For this review, take the finished solid that the model builds, in its own axes (mm). Face numbers are marked on the shaded views. A direction names the side the tool comes from. Coordinates: 2 decimals unless noted, no trailing zeros. Loops run counter-clockwise (first coordinate to the right, second up) from the corner with the lowest first, then second, coordinate; pieces in that order, holes last. Notation, with made-up numbers: M -40,-22 L -18,-22 A23 ccw -18,-3 Z; hole C 80.25,-25 d3. An arc over 180 degrees is marked long. Put each result on its own line as item: value.
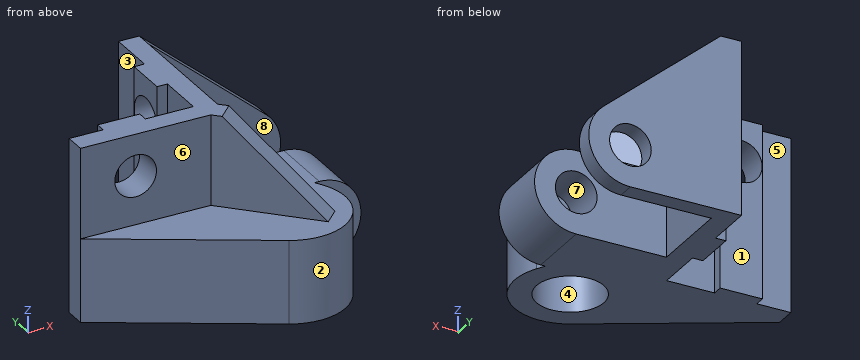
```python
from build123d import *

# Parameters (mm, degrees)
BOSS_EXTRUDE1_DEPTH      = 25
SKETCH2_R                = 3
CUT_EXTRUDE1_DEPTH       = 15
SKETCH3_R                = 3
CUT_EXTRUDE2_DEPTH       = 15
BOSS_EXTRUDE2_DEPTH      = 12
BOSS_EXTRUDE4_DEPTH      = 1.5
SKETCH6_R                = 4.85
CUT_EXTRUDE3_DEPTH       = 9
BOSS_EXTRUDE5_DEPTH      = 2
BOSS_EXTRUDE5_DEPTH_BACK = 0.5
BOSS_EXTRUDE6_START      = -12.37
BOSS_EXTRUDE6_DEPTH      = 9.40874333
BOSS_EXTRUDE7_DEPTH      = 2.5
SKETCH10_R               = 3
CUT_EXTRUDE4_DEPTH       = 21


with BuildPart() as part:
    # Sketch1 → Boss-Extrude1 (new body)
    with BuildSketch(Plane.XY):
        Polygon((227.088719843, 62.282971172), (227.088719843, 57.379571172), (225.590119843, 57.379571172), (225.590119843, 51.299571172), (227.088719843, 51.299571172), (227.088719843, 44.429550862), (220.178702595, 44.429550862), (220.178702595, 45.917195068), (214.098687419, 45.917195068), (214.098687419, 44.429550862), (209.19527518, 44.429550862), (209.19527518, 41.429550862), (230.088719843, 41.429550862), (230.088719843, 62.282971172), align=None)
    extrude(amount=-BOSS_EXTRUDE1_DEPTH)

    # Sketch2 → Cut-Extrude1 (cut)
    with BuildSketch(Plane(origin=(230.088719843, 0, 0), x_dir=(0, 0, -1), z_dir=(1, 0, 0))):
        with Locations((6, 54.339571172)):
            Circle(SKETCH2_R)
    extrude(amount=-CUT_EXTRUDE1_DEPTH, mode=Mode.SUBTRACT)

    # Sketch3 → Cut-Extrude2 (cut)
    with BuildSketch(Plane.XZ.offset(-41.429550862)):
        with Locations((217.138695007, -6)):
            Circle(SKETCH3_R)
    extrude(amount=-CUT_EXTRUDE2_DEPTH, mode=Mode.SUBTRACT)

    # Sketch4 → Boss-Extrude2 (add)
    with BuildSketch(Plane(origin=(0, 0, -25), x_dir=(-1, 0, 0), z_dir=(0, 0, -1))):
        with BuildLine():
            Line((-237.925828106, 48.429550862), (-243.051733392, 39.368642422))
            ThreePointArc((-243.051733392, 39.368642422), (-241.747687926, 29.774811236), (-232.154834185, 28.463594817))
            Line((-232.154834185, 28.463594817), (-209.19527518, 41.429550862))
            Line((-209.19527518, 41.429550862), (-230.088719843, 41.429550862))
            Line((-230.088719843, 41.429550862), (-230.088719843, 48.429550862))
            Line((-230.088719843, 48.429550862), (-237.925828106, 48.429550862))
        make_face()
    extrude(amount=-BOSS_EXTRUDE2_DEPTH)

    # Sketch5 → Boss-Extrude4 (add, symmetric)
    with BuildSketch(Plane(origin=(135.717402312, 135.766641949, 0), x_dir=(0.707235019, -0.70697852, 0), z_dir=(-0.70697852, -0.707235019, 0))):
        Polygon((133.436997596, -13), (147.436997596, -13), (133.436997596, 0), (129.194356979, 0), (129.194356979, -13), align=None)
    extrude(amount=BOSS_EXTRUDE4_DEPTH, both=True)

    # Sketch6 → Cut-Extrude3 (cut)
    with BuildSketch(Plane(origin=(0, 0, -25), x_dir=(-1, 0, 0), z_dir=(0, 0, -1))):
        with Locations((-236.088719843, 35.429550862)):
            Circle(SKETCH6_R)
    extrude(amount=-CUT_EXTRUDE3_DEPTH, mode=Mode.SUBTRACT)

    # Sketch8 → Boss-Extrude5 (add, two sides)
    with BuildSketch(Plane(origin=(0, 62.282971172, 0), x_dir=(-1, 0, 0), z_dir=(0, 1, 0))) as boss_extrude5_sk:
        with BuildLine():
            Line((-227.088719843, -25), (-243.088719843, -25))
            ThreePointArc((-243.088719843, -25), (-249.088719843, -19), (-243.088719843, -13))
            Line((-243.088719843, -13), (-227.088719843, -13))
            Line((-227.088719843, -13), (-227.088719843, -25))
        make_face()
    extrude(amount=BOSS_EXTRUDE5_DEPTH)
    extrude(boss_extrude5_sk.sketch, amount=-BOSS_EXTRUDE5_DEPTH_BACK)

    # Sketch8_2 → Boss-Extrude6 (add)
    with BuildSketch(Plane(origin=(0, 62.282971172, 0), x_dir=(-1, 0, 0), z_dir=(0, 1, 0)).offset(BOSS_EXTRUDE6_START)):
        with BuildLine():
            Line((-227.088719843, -25), (-243.088719843, -25))
            ThreePointArc((-243.088719843, -25), (-249.088719843, -19), (-243.088719843, -13))
            Line((-243.088719843, -13), (-227.088719843, -13))
            Line((-227.088719843, -13), (-227.088719843, -25))
        make_face()
    extrude(amount=-BOSS_EXTRUDE6_DEPTH)

    # Sketch9 → Boss-Extrude7 (add)
    with BuildSketch(Plane(origin=(0, 64.282971172, 0), x_dir=(-1, 0, 0), z_dir=(0, 1, 0))):
        with BuildLine():
            Line((-227.088719843, -13), (-227.088719843, 0))
            Line((-227.088719843, 0), (-230.088719843, 0))
            Line((-230.088719843, 0), (-246.986411594, -14.438421434))
            ThreePointArc((-246.986411594, -14.438421434), (-245.166041268, -13.371080415), (-243.088719843, -13))
            Line((-243.088719843, -13), (-227.088719843, -13))
        make_face()
    extrude(amount=-BOSS_EXTRUDE7_DEPTH)

    # Sketch10 → Cut-Extrude4 (cut)
    with BuildSketch(Plane(origin=(0, 64.282971172, 0), x_dir=(-1, 0, 0), z_dir=(0, 1, 0))):
        with Locations((-243.088719843, -19)):
            Circle(SKETCH10_R)
    extrude(amount=-CUT_EXTRUDE4_DEPTH, mode=Mode.SUBTRACT)


solid = part.part
```
(1) Tool access review of the marked faces 4, 5, 6, 7 and 8: name each direction out of +Z, -Z, +X, -X, +Y, -Y from which nothing blocks a thin tool from reaching the whole face with its end or side.
Determined:
face 4: -Z
face 5: +Z, -Z, -X, +Y
face 6: +Z, -X, -Y
face 7: +Y
face 8: +Z, -Z, +X
(2) Add section D-D (z = -23.5). Write out the cut boundary in (x, y), plus the area to 3 significant figures.
Determined:
outline: M 209.2,41.43 L 232.15,28.46 A8 ccw 243.05,39.37 L 242.41,40.5 L 247.06,40.5 L 247.06,49.91 L 230.09,49.91 L 230.09,61.78 L 247.06,61.78 L 247.06,64.28 L 227.09,64.28 L 227.09,57.38 L 225.59,57.38 L 225.59,51.3 L 227.09,51.3 L 227.09,44.43 L 220.18,44.43 L 220.18,45.92 L 214.1,45.92 L 214.1,44.43 L 209.2,44.43 Z; hole C 236.09,35.43 d9.7
area: 554 mm^2
(3) Draft analysis for pull direction Y (two halves, no side actions). For the marked faces 1, 2 and 3, state which applies: +Y half, -Y half, draft (parallel to the pull), parting line (faces both ways), or undercut.
Determined:
face 1: +Y half
face 2: undercut
face 3: draft
(4) Wall thickness on line 1 along Y through (x, z) = (238.5, -20); line 2 along Y through (x, z) = (218, -10.5); line 3 along X through (y, z) = (60, -7.25): over which ranges is each line inside the solid? List them lowest first. Write a range as [from, to].
Determined:
line 1: y = [27.8, 31.22], [39.64, 49.91], [61.78, 64.28]
line 2: y = [41.43, 45.92]
line 3: x = [227.09, 230.09]
(5) Add section B-B (y = 52). Write out the cut boundary in (x, z), plus the area to 3 significant figures.
Determined:
outline: M 225.59,-25 L 230.09,-25 L 230.09,-7.88 L 225.59,-7.88 Z; M 225.59,-4.12 L 230.09,-4.12 L 230.09,0 L 225.59,0 Z
area: 95.6 mm^2
(6) Add section A-A (z = -17.5). State how many separate pieces and enclosed holes the cut face has, plus the area to 3 significant figures.
Determined:
separate pieces: 2
enclosed holes: 1
area: 528 mm^2
(7) For pin 1 (6.5 mm diameter, centred on y = 53, z = -7.5, fed in from -X); pin 2 (7.5 mm diameter, centred on x = 245, z = -19, fed in from -Y); pin 3 (6 mm diameter, centred on y = 46.5, z = -11.5, fed in from +X); pin 4 (5.5 mm diameter, centred on x = 217.14, z = -6, fed in from -Y), all flat-tipped, find the tip position at first contact; note any pin that passes through.
Determined:
pin 1: stops at x = 225.59
pin 2: stops at y = 29.32
pin 3: stops at x = 247.06
pin 4: passes through
